from build123d import *

# Parameters (mm, degrees)
SKETCH2_R          = 8
CUT_EXTRUDE1_DEPTH = 517.284805122


with BuildPart() as part:
    # Sketch1 → Revolve1 (revolve)
    with BuildSketch(Plane(origin=(0, 0, 0), x_dir=(0, 0, -1), z_dir=(1, 0, 0)), mode=Mode.PRIVATE) as revolve1_sk:
        Polygon((-365, 19.995973642), (-365, 9.995973642), (0, 9.995973642), (0, 24.995973642), (-317, 24.995973642), (-317, 19.995973642), align=None)
    revolve(revolve1_sk.sketch.rotate(Axis((0, 9.995973642, 0), (0, 1, 0)), 180), axis=Axis((0, 9.995973642, 0), (0, 1, 0)))

    # Sketch2 → Cut-Extrude1 (cut, through all)
    with BuildSketch(Plane(origin=(0, 19.995973642, 0), x_dir=(1, 0, 0), z_dir=(0, 1, 0))):
        with Locations(Location((0, 345, 0), (0, 0, 270))):
            Circle(SKETCH2_R)
        with Locations(Location((132.025784166, 318.738438716, 0), (0, 0, 270))):
            Circle(SKETCH2_R)
        with Locations(Location((243.951839509, 243.951839509, 0), (0, 0, 270))):
            Circle(SKETCH2_R)
        with Locations(Location((318.738438716, 132.025784166, 0), (0, 0, 270))):
            Circle(SKETCH2_R)
        with Locations(Location((345, 0, 0), (0, 0, 270))):
            Circle(SKETCH2_R)
        with Locations(Location((318.738438716, -132.025784166, 0), (0, 0, 270))):
            Circle(SKETCH2_R)
        with Locations(Location((243.951839509, -243.951839509, 0), (0, 0, 270))):
            Circle(SKETCH2_R)
        with Locations(Location((132.025784166, -318.738438716, 0), (0, 0, 270))):
            Circle(SKETCH2_R)
        with Locations(Location((0, -345, 0), (0, 0, 270))):
            Circle(SKETCH2_R)
        with Locations(Location((-132.025784166, -318.738438716, 0), (0, 0, 270))):
            Circle(SKETCH2_R)
        with Locations(Location((-243.951839509, -243.951839509, 0), (0, 0, 270))):
            Circle(SKETCH2_R)
        with Locations(Location((-318.738438716, -132.025784166, 0), (0, 0, 270))):
            Circle(SKETCH2_R)
        with Locations(Location((-345, 0, 0), (0, 0, 270))):
            Circle(SKETCH2_R)
        with Locations(Location((-318.738438716, 132.025784166, 0), (0, 0, 270))):
            Circle(SKETCH2_R)
        with Locations(Location((-243.951839509, 243.951839509, 0), (0, 0, 270))):
            Circle(SKETCH2_R)
        with Locations(Location((-132.025784166, 318.738438716, 0), (0, 0, 270))):
            Circle(SKETCH2_R)
    extrude(amount=-CUT_EXTRUDE1_DEPTH, mode=Mode.SUBTRACT)


solid = part.part
Input: part model. Units: mm. Frame: model coordinates. A direction names the side the tool comes from. Round coordinates to 2 decimals unless told otherwise and drop trailing zeros. Write each loop counter-clockwise with the first axis right and the second up, starting at its lowest first coordinate (ties: lowest second). Pieces come first, ordered by that corner, then holes.
1) Cut plane A-A (z = 156.5). Return the cut outline in (x, y).
2) Cut plane B-B (x = 170). Return the cut outline in (y, z), then the cut area to 3 significant figures.
3) Reachability of faces 5 (the cylindrical face through (236.854, 15.066, -240.26)), 6 (the cylindrical face through (-314.3, 22.5, 41.3)) from +Z, -Z, +X, -X, +Y, -Y: full face, straight path, thin tool, end or side. Return the list, or none.
4) Contact query for flat-ended pins moving along their axis: P1, Ø9.5, axis at x = 0, z = 345, coming from the -Y side; P2, Ø18.5, axis at x = 132.03, z = 318.74, coming from the +Y side; P3, Ø1.5, axis at x = 205, y = 13, coming from the +Z side; P4, Ø4, axis at y = 13, z = 163.5, coming from the +X side. Output: stop coordinate, or through.
5) Cut plane C-C (y = 14.5). Count the separate pieces of the cut face and the enclosed holes in it, then the cut area to 3 significant figures.
6) Draft query along Z for faces 1 (the flat face through (106, 19.996, -299)), 2 (the cylindrical face through (311, 15, 130)), 3 (the cylindrical face through (-109.636, 14.926, -348.145)), 4 (the cylindrical face through (2.4, 15.07, 352.63)). Return one class per face: pulls with the +Z half, pulls with the -Z half, needs draft (parallel to the pull), parting line crosses it, or undercut.
7) Ray query, L1, parallel to Y at x = 334, z = 76; L2, parallel to X at y = 18, z = 87; L3, parallel to Z at x = -186, y = 10.5. Return the intervals inside material, ascending.
Geometry says:
1. outline: (-329.75, 10) - (329.75, 10) - (329.75, 20) - (275.68, 20) - (275.68, 25) - (-275.68, 25) - (-275.68, 20) - (-329.75, 20) - close
2. outline: (10, -322.99) - (20, -322.99) - (20, -267.56) - (25, -267.56) - (25, 267.56) - (20, 267.56) - (20, 322.99) - (10, 322.99) - close
2. area: 9,140 mm2
3. face 5: +Y, -Y
3. face 6: +Y
4. P1: passes through
4. P2: stops at y = 20
4. P3: stops at z = 302.5
4. P4: stops at x = 327.33
5. separate pieces: 1
5. enclosed holes: 16
5. area: 415,000 mm2
6. face 1: needs draft
6. face 2: undercut
6. face 3: parting line crosses it
6. face 4: undercut
7. L1: y = 10 to 20
7. L2: x = -354.48 to 354.48
7. L3: z = -314.05 to 314.05
